Design review of the part built by this model. Coordinates are the model's own, in mm. A direction names the side the tool comes from. Give positions to 0.01 mm unless a question says otherwise; leave off trailing zeros. Order: outer loops, then holes, each group sorted by start corner. A loop starts at its lowest first (then second) coordinate and runs counter-clockwise, first axis right, second up.
```python
from build123d import *

# Parameters (mm, degrees)
SKETCH1_R           = 10.287
BOSS_EXTRUDE1_DEPTH = 3.175
SKETCH3_R           = 4.064
CUT_EXTRUDE1_DEPTH  = 2.38125
FILLET1_R           = 1.000000032
CUT_EXTRUDE2_REACH  = 16.89
SKETCH4_R           = 1.27
CIRPATTERN1_COUNT   = 4
SKETCH5_R           = 6.35
BOSS_EXTRUDE2_DEPTH = 20.32
SKETCH6_W           = 9.652
SKETCH6_H           = 6.35
CUT_EXTRUDE3_DEPTH  = 19.05


with BuildPart() as part:
    # Sketch1 → Boss-Extrude1 (new body)
    with BuildSketch(Plane.XY):
        Circle(SKETCH1_R)
    extrude(amount=BOSS_EXTRUDE1_DEPTH)

    # Sketch3 → Cut-Extrude1 (cut)
    with BuildSketch(Plane(origin=(0, 0, 0), x_dir=(-1, 0, 0), z_dir=(0, 0, -1))):
        Circle(SKETCH3_R)
    extrude(amount=-CUT_EXTRUDE1_DEPTH, mode=Mode.SUBTRACT)

    # Fillet1
    fillet1_edges = [part.edges().sort_by_distance(p)[0] for p in [
        (4.064, 0, 0),
    ]]
    fillet(fillet1_edges, radius=FILLET1_R)

    # Sketch4 → Cut-Extrude2 (cut, up to next)
    with BuildSketch(Plane(origin=(0, 0, 0), x_dir=(-1, 0, 0), z_dir=(0, 0, -1)), mode=Mode.PRIVATE) as cut_extrude2_sk1:
        with Locations((0, 7.874)):
            Circle(SKETCH4_R)
    cut_extrude2_tool1 = extrude(cut_extrude2_sk1.sketch, amount=-CUT_EXTRUDE2_REACH, mode=Mode.PRIVATE) & part.part
    cut_extrude2 = cut_extrude2_tool1.solids().sort_by_distance((0, 7.874, 0))[0]
    add(cut_extrude2, mode=Mode.SUBTRACT)

    # CirPattern1: Cut-Extrude2 ×4 about axis
    cirpattern1_axis = Axis((0, 0, 0), (0, 0, 1))
    for i in range(1, CIRPATTERN1_COUNT):
        add(cut_extrude2.rotate(cirpattern1_axis, i * 360 / CIRPATTERN1_COUNT), mode=Mode.SUBTRACT)

    # Sketch5 → Boss-Extrude2 (add)
    with BuildSketch(Plane.XY.offset(3.175)):
        Circle(SKETCH5_R)
    extrude(amount=BOSS_EXTRUDE2_DEPTH)

    # Sketch6 → Cut-Extrude3 (cut)
    with BuildSketch(Plane.XY.offset(23.495)):
        Rectangle(SKETCH6_W, SKETCH6_H)
    extrude(amount=-CUT_EXTRUDE3_DEPTH, mode=Mode.SUBTRACT)


solid = part.part
```
1. For line 1 along Y through (x, z) = (0, 2.2); line 2 along Z through (x, y) = (-3, 2.5) (3 decimals); line 3 along Z through (x, y) = (-1.5, -6.25) (3 decimals), list the stretches that pass through material, from the lowest coordinate up.
Recorded:
line 1: y = -10.29 to -9.14, -6.6 to -4.06, 4.06 to 6.6, 9.14 to 10.29
line 2: z = 2.381 to 4.445
line 3: z = 0 to 3.175
2. Take a section at C-C (z = 13). State the section outline as (x, y) points (3 decimals).
Recorded:
outline: circle Ø12.7 at (0, 0); hole (-4.826, -3.175) - (4.826, -3.175) - (4.826, 3.175) - (-4.826, 3.175) - close
3. Draft analysis for pull direction Y (two halves, no side actions). For faces 4 (the face through (-5, -2, 0)), 5 (the face through (-1.34, 10.2, 1.57)), 6 (the face through (0, 3.175, 14)), state which applies: pulls with the +Y half, pulls with the -Y half, needs draft (parallel to the pull), parting line crosses it, or undercut.
Recorded:
face 4: needs draft
face 5: parting line crosses it
face 6: undercut
4. For pin 1 (5 mm diameter, centred on y = 1, z = 14, fed in from -X); pin 2 (7.5 mm diameter, centred on x = 0, z = 10.5, fed in from -Y); pin 3 (5 mm diameter, centred on y = -1.5, z = 17.5, fed in from +X), all flat-tipped, find the tip position at first contact; note any pin that passes through.
Recorded:
pin 1: stops at x = -6.35
pin 2: stops at y = -6.35
pin 3: stops at x = 6.35
5. Take a section at D-D (x = -7.25). State the section outline as (y, z) points (3 decimals), then the cut area to 3 significant figures.
Recorded:
outline: (-7.298, 0) - (-1.106, 0) - (-1.106, 3.175) - (-7.298, 3.175) - close; (1.106, 0) - (7.298, 0) - (7.298, 3.175) - (1.106, 3.175) - close
area: 39.3 mm2
6. Take a section at A-A (y = 0). State the section outline as (x, z) points (3 decimals).
Recorded:
outline: (-10.287, 0) - (-9.144, 0) - (-9.144, 3.175) - (-10.287, 3.175) - close; (-6.604, 0) - (-5.064, 0) arc R1 ccw to (-4.064, 1) - (-4.064, 2.381) - (4.064, 2.381) - (4.064, 1) arc R1 ccw to (5.064, 0) - (6.604, 0) - (6.604, 3.175) - (6.35, 3.175) - (6.35, 23.495) - (4.826, 23.495) - (4.826, 4.445) - (-4.826, 4.445) - (-4.826, 23.495) - (-6.35, 23.495) - (-6.35, 3.175) - (-6.604, 3.175) - close; (9.144, 0) - (10.287, 0) - (10.287, 3.175) - (9.144, 3.175) - close
7. Take a section at B-B (x = 0). State the section outline as (y, z) points (3 decimals).
Recorded:
outline: (-10.287, 0) - (-9.144, 0) - (-9.144, 3.175) - (-10.287, 3.175) - close; (-6.604, 0) - (-5.064, 0) arc R1 ccw to (-4.064, 1) - (-4.064, 2.381) - (4.064, 2.381) - (4.064, 1) arc R1 ccw to (5.064, 0) - (6.604, 0) - (6.604, 3.175) - (6.35, 3.175) - (6.35, 23.495) - (3.175, 23.495) - (3.175, 4.445) - (-3.175, 4.445) - (-3.175, 23.495) - (-6.35, 23.495) - (-6.35, 3.175) - (-6.604, 3.175) - close; (9.144, 0) - (10.287, 0) - (10.287, 3.175) - (9.144, 3.175) - close
8. Machinability: for faces 1 (the face through (0.881, -3.967, 1.681)), 2 (the face through (-8.945, -0.683, 1.565)), 3 (the face through (4.826, 0, 14)), which of the approach directions +Z, -Z, +X, -X, +Y, -Y give a long, thin tool a straight path to every point of the face, cutting with its end or side? Answer none if there is none.
Recorded:
face 1: -Z
face 2: +Z, -Z
face 3: +Z
